```python
from build123d import *

# Parameters (mm, degrees)
SM_BASE_FLANGE_1_DEPTH           = 2
SKETCH_7_R                       = 10
SKETCH_7_R_2                     = 2
CUT_EXTRUDE_1_DEPTH              = 50.460967207
SM_EDGE_FLANGE_1_STRIP_W         = 10
SM_EDGE_FLANGE_1_STRIP_H         = 2
SM_EDGE_FLANGE_1_STRIP_CUT_DEPTH = 40
SM_EDGE_FLANGE_1_DEPTH           = 40
CUT_EXTRUDE_2_DEPTH              = 89.761563758


# Sheet-metal steps are written as plain solids
with BuildPart() as part:
    # Sketch 1 → 基体-法兰1 (new body)
    with BuildSketch(Plane.XY):
        with BuildLine():
            Line((-31.41539068, 9.119339374), (18.58460932, 9.119339374))
            ThreePointArc((18.58460932, 9.119339374), (38.58460932, -10.880660626), (18.58460932, -30.880660626))
            Line((18.58460932, -30.880660626), (-31.41539068, -30.880660626))
            Line((-31.41539068, -30.880660626), (-31.41539068, 9.119339374))
        make_face()
    extrude(amount=-SM_BASE_FLANGE_1_DEPTH)

    # 草图7 → 切除-拉伸1 (cut, through all)
    with BuildSketch(Plane.XY):
        with Locations((18.58460932, -10.880660626)):
            Circle(SKETCH_7_R)
        with Locations((2.928014356, -10.880660626)):
            Circle(SKETCH_7_R_2)
        with Locations((26.412906802, 2.67834835)):
            Circle(SKETCH_7_R_2)
        with Locations((26.412906802, -24.439669602)):
            Circle(SKETCH_7_R_2)
    extrude(amount=-CUT_EXTRUDE_1_DEPTH, mode=Mode.SUBTRACT)

    # 边线-法兰1 strip (across the edge) → 边线-法兰1 strip cut (cut)
    with BuildSketch(Plane(origin=(-31.41539068, 9.119339374, 0), x_dir=(1, 0, 0), z_dir=(0, -1, 0))):
        with Locations((-4, -1)):
            Rectangle(SM_EDGE_FLANGE_1_STRIP_W, SM_EDGE_FLANGE_1_STRIP_H)
    extrude(amount=SM_EDGE_FLANGE_1_STRIP_CUT_DEPTH, mode=Mode.SUBTRACT)

    # 边线-法兰1 section (across the edge) → 边线-法兰1 (add)
    with BuildSketch(Plane(origin=(-31.41539068, 9.119339374, 0), x_dir=(1, 0, 0), z_dir=(0, -1, 0))):
        with BuildLine():
            Line((-2, 1), (-2, 45))
            Line((-2, 45), (0, 45))
            Line((0, 45), (0, 1))
            ThreePointArc((0, 1), (0.292893219, 0.292893219), (1, 0))
            Line((1, 0), (1, -2))
            ThreePointArc((1, -2), (-1.121320344, -1.121320344), (-2, 1))
        make_face()
    extrude(amount=SM_EDGE_FLANGE_1_DEPTH)

    # 草图11 → 切除-拉伸2 (cut, through all)
    with BuildSketch(Plane(origin=(-31.41539068, 0, 0), x_dir=(0, 0, -1), z_dir=(1, 0, 0))):
        with BuildLine():
            Line((-39, 6.119339374), (-23.313924612, 6.119339374))
            ThreePointArc((-23.313924612, 6.119339374), (-21.313924612, 4.119339374), (-23.313924612, 2.119339374))
            Line((-23.313924612, 2.119339374), (-39, 2.119339374))
            ThreePointArc((-39, 2.119339374), (-41, 4.119339374), (-39, 6.119339374))
        make_face()
        with BuildLine():
            Line((-39, -27.880660626), (-23.313924612, -27.880660626))
            ThreePointArc((-23.313924612, -27.880660626), (-21.313924612, -25.880660626), (-23.313924612, -23.880660626))
            Line((-23.313924612, -23.880660626), (-39, -23.880660626))
            ThreePointArc((-39, -23.880660626), (-41, -25.880660626), (-39, -27.880660626))
        make_face()
    extrude(amount=-CUT_EXTRUDE_2_DEPTH, mode=Mode.SUBTRACT)


solid = part.part
```
Model file for the job. Use its own axes, mm. A direction names the side the tool comes from. Coordinates: 2 decimals unless noted, no trailing zeros. Write each loop counter-clockwise with the first axis right and the second up, starting at its lowest first coordinate (ties: lowest second). Pieces come first, ordered by that corner, then holes. Notation, with made-up numbers: (30, 82) - (80, 82) arc R32 cw to (80, 113) - close; hole circle Ø3 at (5, -19.5). An arc over 180 degrees is marked (long way). Use a Markdown table: item, result. Add a question column.
Item 1: Band-saw the part on B-B, the plane y = -3.5. Write the cut outline in (x, z), and give its area (3 significant figures).
Item 2: Band-saw the part on A-A, the plane z = 35. Write the cut outline in (x, y), and give its area (3 significant figures).
Item 3: Band-saw the part on D-D, the plane x = -6. Write the cut outline in (y, z), and give its area (3 significant figures).
Item 4: Band-saw the part on C-C, the plane y = -12. Write the cut outline in (x, z).
Item 5: Two-plate mould, pull along X, no slides. Class faces 4 (the face through (4, -9.19, -0.99)), 5 (the face through (-32.401, -25.925, 21.314)), 6 (the face through (-32.513, -10.601, -1.145)): pulls with the +X half, pulls with the -X half, needs draft (parallel to the pull), parting line crosses it, or undercut.
Item 6: Drill centre lines: line 1 along X through (y, z) = (-21, 37); line 2 along Z through (x, y) = (-1, -22.5). Where is each one in solid material? Low to high.
Item 7: Drop flat-ended pins along their axis: pin 1 (4 mm diameter, centred on x = -4, y = -18, fed in from +Z); pin 2 (10 mm diameter, centred on x = 18, y = -15.5, fed in from -Z); pin 3 (10 mm diameter, centred on y = -9, z = 33, fed in from +X). Give the stop position or say it passes through.
Item 8: 3-axis set-ups, long thin cutter, end or side, ignore diameter. For faces 1 (the face through (-32, -11, 45)), 2 (the face through (-31.415, -11, 23)), 3 (the face through (-32, -23.881, 31)): which of +Z, -Z, +X, -X, +Y, -Y reach the whole face in a straight line?
A:
| question | item | result |
|---|---|---|
| 1 | outline | (-33.42, 1) arc R3 ccw to (-30.42, -2) - (11.84, -2) - (11.84, 0) - (-30.42, 0) arc R1 cw to (-31.42, 1) - (-31.42, 45) - (-33.42, 45) - close; (25.33, -2) - (37.17, -2) - (37.17, 0) - (25.33, 0) - close |
| 1 | area | 202 mm² |
| 2 | outline | (-33.42, -30.88) - (-31.42, -30.88) - (-31.42, -27.88) - (-33.42, -27.88) - close; (-33.42, -23.88) - (-31.42, -23.88) - (-31.42, 2.12) - (-33.42, 2.12) - close; (-33.42, 6.12) - (-31.42, 6.12) - (-31.42, 9.12) - (-33.42, 9.12) - close |
| 2 | area | 64.0 mm² |
| 3 | outline | (-30.88, -2) - (9.12, -2) - (9.12, 0) - (-30.88, 0) - close |
| 3 | area | 80.0 mm² |
| 4 | outline | (-33.42, 1) arc R3 ccw to (-30.42, -2) - (1.27, -2) - (1.27, 0) - (-30.42, 0) arc R1 cw to (-31.42, 1) - (-31.42, 45) - (-33.42, 45) - close; (4.59, -2) - (8.65, -2) - (8.65, 0) - (4.59, 0) - close; (28.52, -2) - (38.55, -2) - (38.55, 0) - (28.52, 0) - close |
| 5 | face 4 | undercut |
| 5 | face 5 | needs draft |
| 5 | face 6 | pulls with the -X half |
| 6 | line 1 | x = -33.42 to -31.42 |
| 6 | line 2 | z = -2 to 0 |
| 7 | pin 1 | stops at z = 0 |
| 7 | pin 2 | passes through |
| 7 | pin 3 | stops at x = -31.42 |
| 8 | face 1 | +Z, +X, -X, +Y, -Y |
| 8 | face 2 | +Z, +X, +Y, -Y |
| 8 | face 3 | +X, -X |
